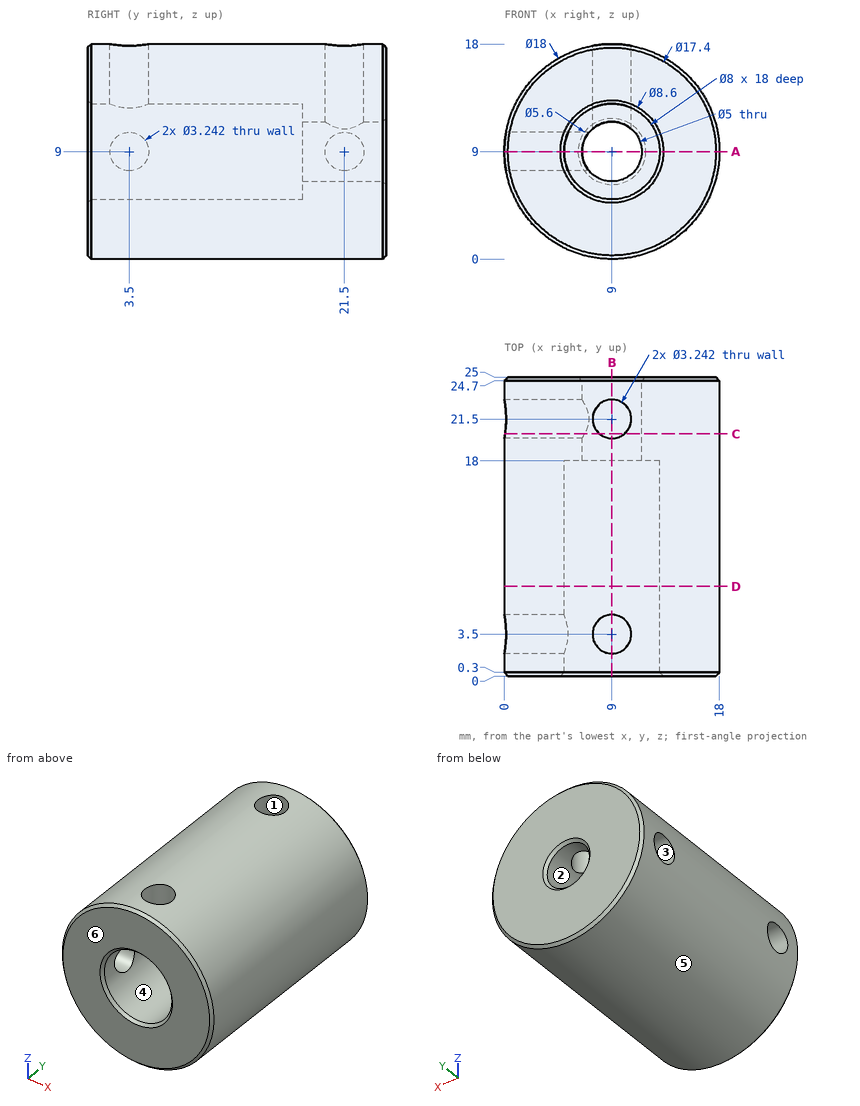
Design review of the part shown in the three views and the two pictorial views. Dimensions are in mm from the part's minimum x, y and z. A direction names the side the tool comes from. Round coordinates to 2 decimals unless told otherwise and drop trailing zeros. Order: outer loops, then holes, each group sorted by start corner. A loop starts at its lowest first (then second) coordinate and runs counter-clockwise, first axis right, second up. Notation, with made-up numbers: (-21, 17.5) -> (-13, 17.5) arc R23 cw to (-13, 45.5) -> close; hole circle Ø4 at (-12, 80). An arc over 180 degrees is marked (long way). Write item = value, one per line. Start each with the question number.
1) Take a section at C-C on y = 20.25. State the section outline as (x, z) points.
2) To check wall thickness, follow line 1 (Y direction, x = 9, z = 16.25); line 2 (Z direction, x = 9, y = 23.75); line 3 (Z direction, x = 9, y = 14). State the ranges of each line that lie inside material, in increasing order. Write a range as from..to.
3) Tool access review of the marked faces 1, 2 and 3: name each direction out of +Z, -Z, +X, -X, +Y, -Y from which nothing blocks a thin tool from reaching the whole face with its end or side.
4) The part is to be moulded in two halves that separate along Z. For the marked faces 4, 5 and 6, say which applies: +Z half, -Z half, draft (parallel to the pull), parting line (faces both ways), or undercut.
5) Take a section at B-B on x = 9. State the section outline as (y, z) points.
6) Insertion check: pin 1 (2.5 mm diameter, centred on x = 10, z = 9, fed in from -Y); pin 2 (1.5 mm diameter, centred on x = 6, y = 7, fed in from -Z); pin 3 (1 mm diameter, centred on y = 11.5, z = 11.5, fed in from -X). Each pin has a flat end and moves straight along its axis. Give the tip position at first contact, or say it passes through.
7) Take a section at A-A on z = 9. State the section outline as (x, y) points.
8) Take a section at D-D on y = 7.5. State the section outline as (x, z) points, plus the area to 3 significant figures.
Verdict:
q1.outline = (0.06, 7.97) arc R9 ccw (long way) to (10.03, 17.94) -> (10.03, 11.28) arc R2.5 cw (long way) to (6.72, 7.97) -> close; (0.06, 10.03) -> (6.72, 10.03) arc R2.5 cw to (7.97, 11.28) -> (7.97, 17.94) arc R9 ccw to start
q2.line_1 = 0..1.88, 5.12..19.88, 23.12..25
q2.line_2 = 0..6.5, 11.5..18
q2.line_3 = 0..5, 13..18
q3.face_1 = +Z
q3.face_2 = +Y, -Y
q3.face_3 = -X
q4.face_4 = undercut
q4.face_5 = parting line
q4.face_6 = draft
q5.outline = (0, 0.3) -> (0.3, 0) -> (24.7, 0) -> (25, 0.3) -> (25, 6.2) -> (24.7, 6.5) -> (18, 6.5) -> (18, 5) -> (0.3, 5) -> (0, 4.7) -> close; (0, 13.3) -> (0.3, 13) -> (1.88, 13) -> (1.88, 18) -> (0.3, 18) -> (0, 17.7) -> close; (5.12, 13) -> (18, 13) -> (18, 11.5) -> (19.88, 11.5) -> (19.88, 18) -> (5.12, 18) -> close; (23.12, 11.5) -> (24.7, 11.5) -> (25, 11.8) -> (25, 17.7) -> (24.7, 18) -> (23.12, 18) -> close
q6.pin_1 = through
q6.pin_2 = 0.29
q6.pin_3 = 0.23
q7.outline = (0, 0.3) -> (0.3, 0) -> (4.7, 0) -> (5, 0.3) -> (5, 1.88) -> (0, 1.88) -> close; (0, 5.12) -> (5, 5.12) -> (5, 18) -> (6.5, 18) -> (6.5, 19.88) -> (0, 19.88) -> close; (0, 23.12) -> (6.5, 23.12) -> (6.5, 24.7) -> (6.2, 25) -> (0.3, 25) -> (0, 24.7) -> close; (11.5, 18) -> (13, 18) -> (13, 0.3) -> (13.3, 0) -> (17.7, 0) -> (18, 0.3) -> (18, 24.7) -> (17.7, 25) -> (11.8, 25) -> (11.5, 24.7) -> close
q8.outline = circle Ø18 at (9, 9); hole circle Ø8 at (9, 9)
q8.area = 204 mm2
